from build123d import *

# Parameters (mm, degrees)
ESBO_O1_W                = 45
ESBO_O1_H                = 20
ESBO_O1_R                = 2
ESBO_O1_R_2              = 1.75
RESSALTO_EXTRUS_O1_DEPTH = 3
FILETE1_R                = 10


with BuildPart() as part:
    # Esboço1 → Ressalto-extrusão1 (new body)
    with BuildSketch(Plane.XY):
        Rectangle(ESBO_O1_W, ESBO_O1_H)
        with Locations((-16.5, 0)):
            Circle(ESBO_O1_R, mode=Mode.SUBTRACT)
        with Locations((-4.5, 0)):
            Circle(ESBO_O1_R, mode=Mode.SUBTRACT)
        with Locations((12.5, 0)):
            Circle(ESBO_O1_R_2, mode=Mode.SUBTRACT)
    extrude(amount=RESSALTO_EXTRUS_O1_DEPTH)

    # Filete1
    filete1_edges = [part.edges().sort_by_distance(p)[0] for p in [
        (22.5, -10, 1.5),
        (22.5, 10, 1.5),
    ]]
    fillet(filete1_edges, radius=FILETE1_R - 0.0001)  # a hair under: the kernel refuses the full size


solid = part.part
Model file for the job. Use its own axes, mm. Coordinates: 2 decimals unless noted, no trailing zeros. Write each loop counter-clockwise with the first axis right and the second up, starting at its lowest first coordinate (ties: lowest second). Pieces come first, ordered by that corner, then holes. Notation, with made-up numbers: (-35.75, -35) -> (-10.75, -35) arc R19 ccw to (-10.75, -26) -> close; hole circle Ø6 at (89, 50.5). An arc over 180 degrees is marked (long way). One line per item, written item: value. Start each with the question number.
1) Pull direction Y, two halves, no side cores. Call faces 1 (the face through (19.49, 7.15, 1.52)), 2 (the face through (0, 0, 3)), 3 (the face through (19.49, -7.15, 1.52)), 4 (the face through (14.169, 0.526, 1.479)): +Y half, -Y half, draft (parallel to the pull), parting line (faces both ways), or undercut.
2) Probe probe 1 along Y at (x, z) = (12.5, 0.8); probe 2 along Y at (x, z) = (-4.5, 0.7); probe 3 along X at (y, z) = (0.75, 2.7). List the from-to ranges inside material, lowest first.
3) Slice it at B-B on x = -4.5. Write the cut outline in (y, z), then the cut area to 3 significant figures.
4) Slice it at D-D on x = 16. Write the cut outline in (y, z).
5) Slice it at C-C on y = -0.5. Write the cut outline in (x, z).
6) Slice it at A-A on z = 1. Count the separate pieces of the cut face and the enclosed holes in it, then the cut area to 3 significant figures.
Answers follow:
1. face 1: +Y half
1. face 2: draft
1. face 3: -Y half
1. face 4: undercut
2. probe 1: -10 to -1.75, 1.75 to 10
2. probe 2: -10 to -2, 2 to 10
2. probe 3: -22.5 to -18.35, -14.65 to -6.35, -2.65 to 10.92, 14.08 to 22.47
3. outline: (-10, 0) -> (-2, 0) -> (-2, 3) -> (-10, 3) -> close; (2, 0) -> (10, 0) -> (10, 3) -> (2, 3) -> close
3. area: 48.0 mm2
4. outline: (-9.37, 0) -> (9.37, 0) -> (9.37, 3) -> (-9.37, 3) -> close
5. outline: (-22.5, 0) -> (-18.44, 0) -> (-18.44, 3) -> (-22.5, 3) -> close; (-14.56, 0) -> (-6.44, 0) -> (-6.44, 3) -> (-14.56, 3) -> close; (-2.56, 0) -> (10.82, 0) -> (10.82, 3) -> (-2.56, 3) -> close; (14.18, 0) -> (22.49, 0) -> (22.49, 3) -> (14.18, 3) -> close
6. separate pieces: 1
6. enclosed holes: 3
6. area: 822 mm2
